Geometry: see drawing. Coordinates: mm, zero at the bounding-box minimum. Coordinates: 2 decimals unless noted, no trailing zeros. Write each loop counter-clockwise with the first axis right and the second up, starting at its lowest first coordinate (ties: lowest second). Pieces come first, ordered by that corner, then holes. Notation, with made-up numbers: (18, 60) - (50, 60) arc R15 ccw to (50, 88) - close; hole circle Ø7 at (58, 15). An arc over 180 degrees is marked (long way). One line per question, with ' | ' between items. Start each with the question number.
1) Section query D-D on x = 57. Return loops of the section in (y, z) (3 decimals), and give its area (3 significant figures).
2) Section query A-A on y = 40. Return loops of the section in (x, z).
3) First-contact query: P1, Ø3, axis at x = 76, y = 40, coming from the -Z side; P2, Ø2, axis at x = 52.5, z = 3, coming from the -Y side; P3, Ø1.5, axis at x = 49, z = 2, coming from the -Y side; P4, Ø3, axis at y = 23.5, z = 1, coming from the +X side. Flat tips, straight axial feed; report the tip coordinate or a pass-through.
4) Section query C-C on z = 4.05. Return loops of the section in (x, y), and give its area (3 significant figures).
5) Draft query along Y for the marked faces 1, 2 and 3. Return one class per face: released by +Y, released by -Y, zero draft, split by the parting line, or undercut.
6) Line query: line 1 (Y direction, x = 40, z = 3.75); line 2 (Y direction, x = 22.5, z = 4); line 3 (X direction, y = 76, z = 2.7). Output: solid intervals per line, ascending.
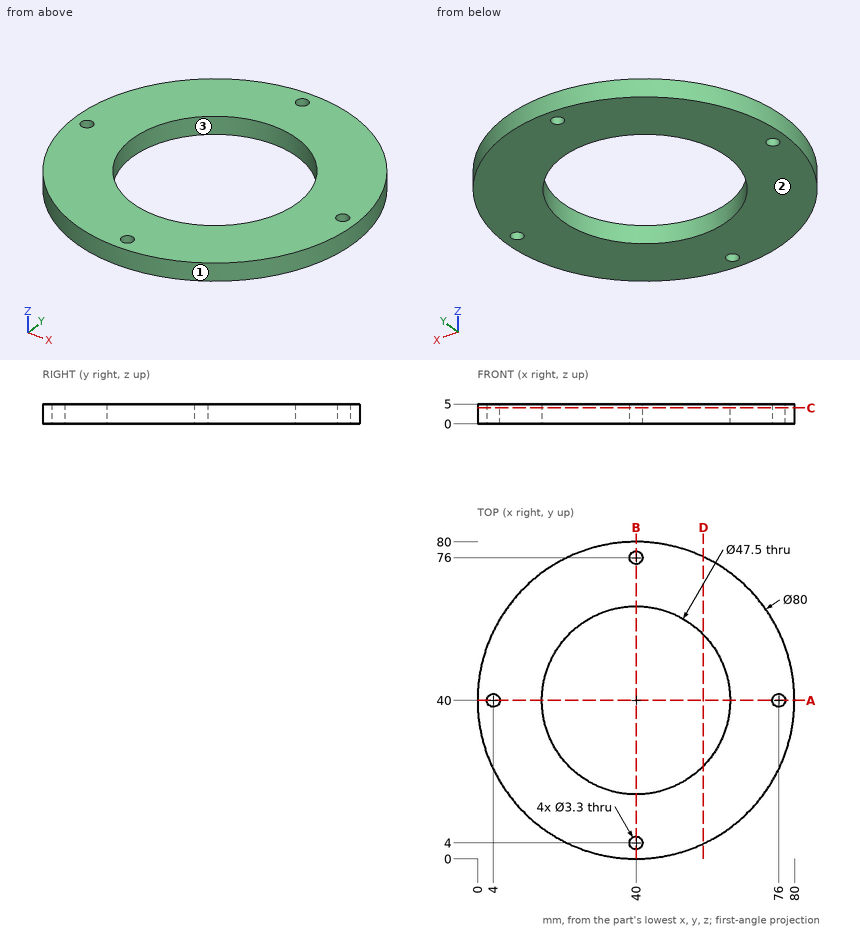
Answer key:
1) outline: (3.792, 0) - (23.415, 0) - (23.415, 5) - (3.792, 5) - close; (56.585, 0) - (76.208, 0) - (76.208, 5) - (56.585, 5) - close | area: 196 mm²
2) outline: (0, 0) - (2.35, 0) - (2.35, 5) - (0, 5) - close; (5.65, 0) - (16.25, 0) - (16.25, 5) - (5.65, 5) - close; (63.75, 0) - (74.35, 0) - (74.35, 5) - (63.75, 5) - close; (77.65, 0) - (80, 0) - (80, 5) - (77.65, 5) - close
3) P1: through | P2: y = 1.69 | P3: y = 0.86 | P4: x = 77.08
4) outline: circle Ø80 at (40, 40); hole circle Ø3.3 at (4, 40); hole circle Ø47.5 at (40, 40); hole circle Ø3.3 at (40, 4); hole circle Ø3.3 at (40, 76); hole circle Ø3.3 at (76, 40) | area: 3,220 mm²
5) face 1: split by the parting line | face 2: zero draft | face 3: undercut
6) line 1: 0 to 2.35, 5.65 to 16.25, 63.75 to 74.35, 77.65 to 80 | line 2: 4.03 to 23.94, 56.06 to 75.97 | line 3: 22.56 to 38.35, 41.65 to 57.44
